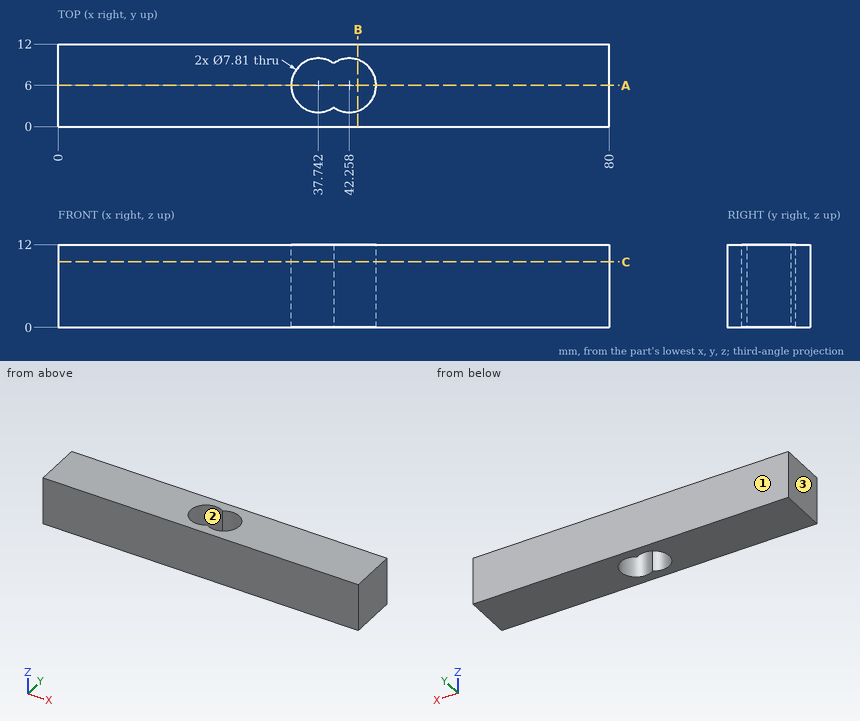
Study the drawing (mm; zero at the part's minimum x, y, z) and answer. Coordinates: 2 decimals unless noted, no trailing zeros. Write each loop counter-clockwise with the first axis right and the second up, starting at its lowest first coordinate (ties: lowest second). Pieces come first, ordered by that corner, then holes. Notation, with made-up numbers: (88, 13.25) -> (126, 13.25) arc R16 cw to (126, 32.25) -> close; hole circle Ø9 at (-26.75, 66.5). An arc over 180 degrees is marked (long way). Write item = value, one per line.
(1) For a pull along Y with two mould halves and no side action, classify the marked faces 1, 2 and 3 as +Y half, -Y half, draft (parallel to the pull), parting line (faces both ways), or undercut.
From the geometry:
face_1 = +Y half
face_2 = undercut
face_3 = draft
(2) Section C-C on z = 9.5 is taken. Write down the section's boundary in (x, y) (1 decimal).
From the geometry:
outline = (0, 0) -> (80, 0) -> (80, 12) -> (0, 12) -> close; hole (40, 2.8) arc R3.9 ccw (long way) to (40, 9.2) arc R3.9 ccw (long way) to start
(3) Section B-B on x = 43.5 is taken. Write down the section's boundary in (y, z).
From the geometry:
outline = (0, 0) -> (2.3, 0) -> (2.3, 12) -> (0, 12) -> close; (9.7, 0) -> (12, 0) -> (12, 12) -> (9.7, 12) -> close
(4) Given pin 1 Ø3 at (y, z) = (5, 4.5) entering from -X; pin 2 Ø6 at (x, y) = (42.26, 6) entering from -Z, each flat-ended and moving along its own axis, determine where each tip first touches the part or whether it passes through.
From the geometry:
pin_1 = 0
pin_2 = through
(5) Straight lines are drawn through the part: L1, parallel to Y at x = 37.5, z = 2.75; L2, parallel to Y at x = 45.5, z = 4.5 (1 decimal); L3, parallel to X at y = 2.75, z = 2.5 (1 decimal). For each, find the intervals that lie inside material, in ascending order. Write a range as from..to.
From the geometry:
L1 = 0..2.1, 9.9..12
L2 = 0..3.8, 8.2..12
L3 = 0..35.6, 39.9..40.1, 44.4..80
(6) Section A-A on y = 6 is taken. Write down the section's boundary in (x, z), plus the area to 3 significant figures.
From the geometry:
outline = (0, 0) -> (33.84, 0) -> (33.84, 12) -> (0, 12) -> close; (46.16, 0) -> (80, 0) -> (80, 12) -> (46.16, 12) -> close
area = 812 mm2
